Build history of the part. All positions in model axes, mm. Coordinates: 2 decimals unless noted, no trailing zeros. Loops run counter-clockwise (first coordinate to the right, second up) from the corner with the lowest first, then second, coordinate; pieces in that order, holes last.
(1) Slice it at C-C (x = 0). Give the cut face in (y, z), and give its area (3 significant figures).
(2) Slice it at D-D (y = -4). Give the cut face in (x, z).
(3) Wall check: L1, parallel to X at y = -8.5, z = 2.1; L2, parallel to Y at x = 1, z = 1.7; L3, parallel to X at y = -7, z = 2.6. Give the ranges that are in metal, low to high.
(4) Two-plate mould, pull along X, no slides. Class faces 1 (the face through (14, 0, 1)), 2 (the face through (-9.363, -0.729, 1.479)), 3 (the face through (0, 0, 0)): pulls with the +X half, pulls with the -X half, needs draft (parallel to the pull), parting line crosses it, or undercut.
(5) Slice it at A-A (y = 2). Give the cut face in (x, z).
(6) Slice it at B-B (z = 1.25). Give the number of separate pieces and of enclosed holes in the cut face, and give its area (3 significant figures).
(7) Flat gauge pins, fed straight in: P1, Ø1.5, axis at x = 10, z = 0.5, coming from the +Y side; P2, Ø2.5, axis at x = 5.51, y = -9.23, coming from the +Z side; P3, Ø1, axis at x = 6, z = 1, coming from the +Y side. Where does each tip first touch, or does it go through?
from build123d import *

# Parameters (mm, degrees)
ESQUISSE1_R        = 18
ESQUISSE1_R_2      = 1.5
BOSS_EXTRU_1_DEPTH = 3


with BuildPart() as part:
    # Esquisse1 → Boss.-Extru.1 (new body)
    with BuildSketch(Plane.XY):
        Circle(ESQUISSE1_R)
        with Locations((5.240453276, 9.386167986)):
            Circle(ESQUISSE1_R_2, mode=Mode.SUBTRACT)
        with Locations((5.508433282, -9.231449657)):
            Circle(ESQUISSE1_R_2, mode=Mode.SUBTRACT)
        with Locations((-10.748886558, -0.154718329)):
            Circle(ESQUISSE1_R_2, mode=Mode.SUBTRACT)
        with BuildLine():
            Line((-11.072133243, -3.407490345), (-1.716682497, -3.409655851))
            Line((-1.716682497, -3.409655851), (2.776978064, -10.990617044))
            ThreePointArc((2.776978064, -10.990617044), (2.840789334, -11.103330491), (2.909041031, -11.213411848))
            ThreePointArc((2.909041031, -11.213411848), (3.02444637, -12.90884018), (1.646159643, -13.902883098))
            ThreePointArc((1.646159643, -13.902883098), (-6.824776359, -12.22384668), (-12.698957381, -5.893766319))
            ThreePointArc((-12.698957381, -5.893766319), (-12.575965538, -4.198871447), (-11.072133243, -3.407490345))
        make_face(mode=Mode.SUBTRACT)
        with BuildLine():
            Line((-11.165620039, 3.087402491), (-2.050122008, 3.087402491))
            Line((-2.050122008, 3.087402491), (2.58509342, 11.292493835))
            ThreePointArc((2.58509342, 11.292493835), (2.651653429, 12.990541357), (1.245327334, 13.944502853))
            ThreePointArc((1.245327334, 13.944502853), (-7.173773577, 12.022353042), (-12.86332977, 5.525825479))
            ThreePointArc((-12.86332977, 5.525825479), (-12.691606715, 3.835172702), (-11.165620039, 3.087402491))
        make_face(mode=Mode.SUBTRACT)
        with BuildLine():
            Line((8.487039823, -7.88500349), (3.740322398, 0.12713591))
            Line((3.740322398, 0.12713591), (8.256579008, 8.126009358))
            ThreePointArc((8.256579008, 8.126009358), (9.667160345, 9.073667479), (11.217170127, 8.377057619))
            ThreePointArc((11.217170127, 8.377057619), (13.998549936, 0.201493638), (11.453630047, -8.050736534))
            ThreePointArc((11.453630047, -8.050736534), (9.92431211, -8.79166991), (8.487039823, -7.88500349))
        make_face(mode=Mode.SUBTRACT)
    extrude(amount=BOSS_EXTRU_1_DEPTH)


solid = part.part
Response values:
1. outline: (-18, 0) - (-14, 0) - (-14, 3) - (-18, 3) - close; (-6.31, 0) - (6.72, 0) - (6.72, 3) - (-6.31, 3) - close; (14, 0) - (18, 0) - (18, 3) - (14, 3) - close
1. area: 63.1 mm2
2. outline: (-17.55, 0) - (-12.42, 0) - (-12.42, 3) - (-17.55, 3) - close; (-1.37, 0) - (6.19, 0) - (6.19, 3) - (-1.37, 3) - close; (13.42, 0) - (17.55, 0) - (17.55, 3) - (13.42, 3) - close
3. L1: x = -15.87 to -11.12, 1.3 to 4.2, 6.82 to 9.05, 10.99 to 15.87
3. L2: y = -17.97 to -13.96, -7.99 to 8.49, 13.96 to 17.97
3. L3: x = -16.58 to -12.12, 0.41 to 7.96, 12.12 to 16.58
4. face 1: undercut
4. face 2: undercut
4. face 3: needs draft
5. outline: (-17.89, 0) - (4.8, 0) - (4.8, 3) - (-17.89, 3) - close; (13.86, 0) - (17.89, 0) - (17.89, 3) - (13.86, 3) - close
6. separate pieces: 1
6. enclosed holes: 6
6. area: 642 mm2
7. P1: stops at y = 15.44
7. P2: passes through
7. P3: stops at y = 17.14
